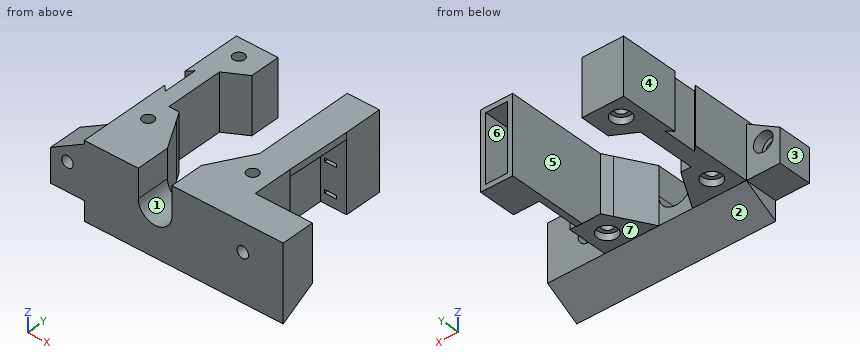
```python
from build123d import *

# Parameters (mm, degrees)
SKETCH1_R                       = 1.7
BOSS_EXTRUDE1_DEPTH             = 16.8
BOSS_EXTRUDE2_DEPTH             = 17
BOSS_EXTRUDE2_DEPTH_BACK        = 42
SKETCH3_W                       = 16.8
SKETCH3_H                       = 10
BOSS_EXTRUDE3_DEPTH             = 10
SKETCH4_R                       = 1.7
CUT_EXTRUDE1_DEPTH              = 11
SKETCH4_3_R                     = 2.9
SKETCH4_3_R_2                   = 1.7
CUT_EXTRUDE2_DEPTH              = 3
CUT_EXTRUDE3_START              = -16.8
SKETCH6_R                       = 2.9
CUT_EXTRUDE3_DEPTH              = 2
CUT_EXTRUDE4_DEPTH              = 11
SKIZZE1_R                       = 5
SCHNITT_LINEAR_AUSTRAGEN1_DEPTH = 53
SCHNITT_LINEAR_AUSTRAGEN2_DEPTH = 17.8
AUFSATZ_LINEAR_AUSTRAGEN1_DEPTH = 16.8
SCHNITT_LINEAR_AUSTRAGEN3_DEPTH = 11
SKETCH13_W                      = 9.5
SKETCH13_H                      = 23
SKETCH13_W_2                    = 6.5
SKETCH13_H_2                    = 20
BOSS_EXTRUDE7_DEPTH             = 10.2
SKETCH14_W                      = 9.5
SKETCH14_H                      = 23
SKETCH14_W_2                    = 3.5
SKETCH14_H_2                    = 1
BOSS_EXTRUDE8_DEPTH             = 1
BOSS_EXTRUDE9_DEPTH             = 2
BOSS_EXTRUDE10_DEPTH            = 1.8
CUT_EXTRUDE10_DEPTH             = 17.8


with BuildPart() as part:
    # Sketch1 → Boss-Extrude1 (new body)
    with BuildSketch(Plane.XY):
        Polygon((-21, 21.339745962), (-21, -20.660254038), (21, -20.660254038), (21, -8.660254038), (15, -8.660254038), (0, -17.320508076), (-15, -8.660254038), (-15, 8.660254038), (-8.626933041, 12.339745962), (-8.626933041, 21.339745962), align=None)
        with Locations((-15.5, -15.160254038)):
            Circle(SKETCH1_R, mode=Mode.SUBTRACT)
        with Locations((15.5, -15.160254038)):
            Circle(SKETCH1_R, mode=Mode.SUBTRACT)
        with Locations((-15.5, 15.839745962)):
            Circle(SKETCH1_R, mode=Mode.SUBTRACT)
    extrude(amount=-BOSS_EXTRUDE1_DEPTH)



with BuildPart() as body_2:
    # Sketch2 → Boss-Extrude2 (new body, two sides)
    with BuildSketch(Plane(origin=(21, 0, 0), x_dir=(0, 0, -1), z_dir=(1, 0, 0))) as boss_extrude2_sk:
        Polygon((0, -20.660254038), (0, -30.660254038), (22.573502692, -30.660254038), (16.8, -20.660254038), align=None)
    extrude(amount=BOSS_EXTRUDE2_DEPTH)
    extrude(boss_extrude2_sk.sketch, amount=-BOSS_EXTRUDE2_DEPTH_BACK)


with BuildPart() as part_1:
    add(part.part)

    add(body_2.part)  # Boss-Extrude3 merges body 2
    # Sketch3 → Boss-Extrude3 (add)
    with BuildSketch(Plane.ZY.offset(21)):
        with Locations((-8.4, -25.660254038)):
            Rectangle(SKETCH3_W, SKETCH3_H)
    extrude(amount=BOSS_EXTRUDE3_DEPTH)

    # Sketch4 → Cut-Extrude1 (cut, through all)
    with BuildSketch(Plane(origin=(0, -20.660254038, 0), x_dir=(1, 0, 0), z_dir=(0, 1, 0))):
        with Locations(Location((-26, 8.4, 0), (0, 0, 270))):  # turned: the seam where the file's is
            Circle(SKETCH4_R)
        with Locations(Location((26, 8.4, 0), (0, 0, 270))):  # turned: the seam where the file's is
            Circle(SKETCH4_R)
    extrude(amount=-CUT_EXTRUDE1_DEPTH, mode=Mode.SUBTRACT)

    # Sketch4_3 → Cut-Extrude2 (cut)
    with BuildSketch(Plane(origin=(0, -20.660254038, 0), x_dir=(1, 0, 0), z_dir=(0, 1, 0))):
        with Locations(Location((-26, 8.4, 0), (0, 0, 270))):  # turned: the seam where the file's is
            Circle(SKETCH4_3_R)
        with Locations(Location((-26, 8.4, 0), (0, 0, 270))):  # turned: the seam where the file's is
            Circle(SKETCH4_3_R_2, mode=Mode.SUBTRACT)
        with Locations(Location((26, 8.4, 0), (0, 0, 90))):  # turned: the seam where the file's is
            Circle(SKETCH4_3_R)
        with Locations(Location((26, 8.4, 0), (0, 0, 270))):  # turned: the seam where the file's is
            Circle(SKETCH4_3_R_2, mode=Mode.SUBTRACT)
    extrude(amount=-CUT_EXTRUDE2_DEPTH, mode=Mode.SUBTRACT)

    # Sketch6 → Cut-Extrude3 (cut)
    with BuildSketch(Plane.XY.offset(CUT_EXTRUDE3_START)):
        with Locations((-15.5, 15.839745962)):
            Circle(SKETCH6_R)
        with Locations((-15.5, -15.160254038)):
            Circle(SKETCH6_R)
        with Locations((15.5, -15.160254038)):
            Circle(SKETCH6_R)
    extrude(amount=CUT_EXTRUDE3_DEPTH, mode=Mode.SUBTRACT)

    # Sketch5 → Cut-Extrude4 (cut, through all)
    with BuildSketch(Plane(origin=(0, -20.660254038, 0), x_dir=(1, 0, 0), z_dir=(0, 1, 0))):
        Polygon((-31, 0), (-31, 6.8), (-21, 1.026497308), (-21, 0), align=None)
    extrude(amount=-CUT_EXTRUDE4_DEPTH, mode=Mode.SUBTRACT)

    # Skizze1 → Schnitt-Linear austragen1 (cut, through all)
    with BuildSketch(Plane.XZ.offset(30.660254038)):
        with Locations((0, -8.5)):
            Circle(SKIZZE1_R)
    extrude(amount=-SCHNITT_LINEAR_AUSTRAGEN1_DEPTH, mode=Mode.SUBTRACT)

    # Skizze2 → Schnitt-Linear austragen2 (cut, through all)
    with BuildSketch(Plane(origin=(0, 0, -16.8), x_dir=(-1, 0, 0), z_dir=(0, 0, -1))):
        Polygon((-5, -20.660254038), (5, -20.660254038), (10.392304845, -11.320508076), (0, -17.320508076), (-10.392304845, -11.320508076), align=None)
    extrude(amount=-SCHNITT_LINEAR_AUSTRAGEN2_DEPTH, mode=Mode.SUBTRACT)

    # Skizze2_3 → Aufsatz-Linear austragen1 (add)
    with BuildSketch(Plane(origin=(0, 0, -16.8), x_dir=(-1, 0, 0), z_dir=(0, 0, -1))):
        Polygon((-15, -8.660254038), (-10.392304845, -11.320508076), (-11.92820323, -8.660254038), align=None)
        Polygon((11.92820323, -8.660254038), (10.392304845, -11.320508076), (15, -8.660254038), align=None)
    extrude(amount=-AUFSATZ_LINEAR_AUSTRAGEN1_DEPTH)

    # Skizze3 → Schnitt-Linear austragen3 (cut, through all)
    with BuildSketch(Plane(origin=(0, -20.660254038, 0), x_dir=(1, 0, 0), z_dir=(0, 1, 0))):
        with BuildLine():
            Line((5, 0), (-5, 0))
            Line((-5, 0), (-5, 8.5))
            ThreePointArc((-5, 8.5), (0, 3.5), (5, 8.5))
            Line((5, 8.5), (5, 0))
        make_face()
    extrude(amount=-SCHNITT_LINEAR_AUSTRAGEN3_DEPTH, mode=Mode.SUBTRACT)



with BuildPart() as body_2_2:
    # Sketch13 → Boss-Extrude7 (new body)
    with BuildSketch(Plane(origin=(0, 21.339745962, 0), x_dir=(1, 0, 0), z_dir=(0, 1, 0))):
        with Locations((16.67820323, 11.5)):
            Rectangle(SKETCH13_W, SKETCH13_H)
        with Locations((16.67820323, 11.5)):
            Rectangle(SKETCH13_W_2, SKETCH13_H_2, mode=Mode.SUBTRACT)
    extrude(amount=-BOSS_EXTRUDE7_DEPTH)

    # Sketch14 → Boss-Extrude8 (add)
    with BuildSketch(Plane.XZ.offset(-11.139745962)):
        with Locations((16.67820323, -11.5)):
            Rectangle(SKETCH14_W, SKETCH14_H)
        with Locations((16.67820323, -19.6)):
            Rectangle(SKETCH14_W_2, SKETCH14_H_2, mode=Mode.SUBTRACT)
        with Locations((16.67820323, -10.8)):
            Rectangle(SKETCH14_W_2, SKETCH14_H_2, mode=Mode.SUBTRACT)
        with Locations((16.67820323, -3.5)):
            Rectangle(SKETCH14_W_2, SKETCH14_H_2, mode=Mode.SUBTRACT)
    extrude(amount=BOSS_EXTRUDE8_DEPTH)


with BuildPart() as part_2:
    add(part_1.part)

    add(body_2_2.part)  # Boss-Extrude9 merges body 2 2
    # Sketch15 → Boss-Extrude9 (add)
    with BuildSketch(Plane.XY):
        Polygon((21.42820323, 10.139745962), (21, -8.660254038), (11.92820323, -8.660254038), (11.92820323, 10.139745962), align=None)
    extrude(amount=-BOSS_EXTRUDE9_DEPTH)

    # Sketch16 → Boss-Extrude10 (add)
    with BuildSketch(Plane.ZY.offset(-11.92820323)):
        Polygon((-2, 10.139745962), (-23, 10.139745962), (-23, -2.460254038), (-16.8, -8.660254038), (-2, -8.660254038), align=None)
    extrude(amount=-BOSS_EXTRUDE10_DEPTH)

    # Sketch18 → Cut-Extrude10 (cut, through all)
    with BuildSketch(Plane(origin=(0, 0, -16.8), x_dir=(-1, 0, 0), z_dir=(0, 0, -1))):
        Polygon((21, 0.339745962), (21, 3.839745962), (19.4, 5.439745962), (19.4, -4.760254038), (21, -3.160254038), align=None)
    extrude(amount=-CUT_EXTRUDE10_DEPTH, mode=Mode.SUBTRACT)


solid = part_2.part
```
Design review of the part built by this model. Coordinates are the model's own, in mm. Face numbers are marked on the shaded views. A direction names the side the tool comes from. Coordinates: 2 decimals unless noted, no trailing zeros. Order: outer loops, then holes, each group sorted by start corner. A loop starts at its lowest first (then second) coordinate and runs counter-clockwise, first axis right, second up.
1) Wall thickness on line 1 along Y through (x, z) = (-15.5, -5); line 2 along Y through (x, z) = (15.5, -4.5); line 3 along X through (y, z) = (13, -7.5): over which ranges is each line inside the solid? List them lowest first.
2) Take a section at D-D, the plane x = 33.5. Give the boundary of the cut face in (y, z).
3) Mouldability with a two-part tool opening along X and no side actions: class the marked faces 1, 2 and 3 as +X half, -X half, draft (parallel to the pull), parting line (faces both ways), or undercut.
4) Take a section at B-B, the plane y = -4. Give the boundary of the cut face in (x, z), and give its area (3 significant figures).
5) Take a section at A-A, the plane x = 26. Give the boundary of the cut face in (y, z), and give its area (3 significant figures).
6) For the marked faces 4, 5, 6 and 7, list the 3-axis set-ups (+Z, -Z, +X, -X, +Y, -Y) from which the entire face can be reached by the end or side of a thin tool; tool diameter is ignored.
7) Take a section at C-C, the plane x = -4. Give the boundary of the cut face in (y, z).
8) Clearance check with flat-ended pins moving along their axes: pin 1 (1.1 mm diameter, centred on y = 10.5, z = -20, fed in from -X); pin 2 (1 mm diameter, centred on y = -11, z = -15, fed in from +X); pin 3 (3 mm diameter, centred on y = -2.5, z = -20, fed in from +X); pin 4 (10 mm diameter, centred on x = -1.5, y = -14, fed in from -Z). State where each tip first meets the part, or that it passes through.
Returned:
1. line 1: y = -30.66 to -16.86, -13.46 to 14.14, 17.54 to 21.34
1. line 2: y = -30.66 to -16.86, -13.46 to -8.66, 10.14 to 11.14
1. line 3: x = -21 to -8.63, 11.93 to 13.43, 19.93 to 21.43
2. outline: (-30.66, -22.57) - (-20.66, -16.8) - (-20.66, 0) - (-30.66, 0) - close
3. face 1: undercut
3. face 2: draft
3. face 3: -X half
4. outline: (-21, -16.8) - (-20.16, -16.8) - (-20.16, 0) - (-21, 0) - close; (-19.4, -16.8) - (-15, -16.8) - (-15, 0) - (-19.4, 0) - close; (11.93, -21.46) - (13.73, -21.46) - (13.73, -2) - (21.11, -2) - (21.11, 0) - (11.93, 0) - close
4. area: 141 mm2
5. outline: (-30.66, -22.57) - (-20.66, -16.8) - (-20.66, -11.3) - (-23.66, -11.3) - (-23.66, -10.1) - (-30.66, -10.1) - close; (-30.66, -6.7) - (-23.66, -6.7) - (-23.66, -5.5) - (-20.66, -5.5) - (-20.66, 0) - (-30.66, 0) - close
5. area: 156 mm2
6. face 4: +Z, -Z, -X, +Y
6. face 5: +Z, -Z, +Y
6. face 6: +Y
6. face 7: -Z, +X, -X
7. outline: (-30.66, -22.57) - (-20.66, -16.8) - (-20.66, -11.5) - (-30.66, -11.5) - close
8. pin 1: stops at x = 11.93
8. pin 2: stops at x = 21
8. pin 3: stops at x = 13.73
8. pin 4: passes through
